The listing builds one solid part. Answer for the finished solid, in the listing's coordinates (mm). A direction names the side the tool comes from. Coordinates: 2 decimals unless noted, no trailing zeros. Order: outer loops, then holes, each group sorted by start corner. A loop starts at its lowest first (then second) coordinate and runs counter-clockwise, first axis right, second up. Notation, with made-up numbers: M -39.5,-7.5 L 10.5,-7.5 A14 cw 10.5,9.5 Z; hole C 19,39.5 d4. An arc over 180 degrees is marked long. One line per item, written item: value. Start each with the question number.
Q1. Straight lines are drawn through the part: line 1 along Z through (x, y) = (0, 18); line 2 along Z through (x, y) = (492.5, -41); line 3 along Y through (x, z) = (147, 80). For each, find the intervals that lie inside material, in ascending order. Write a range as [from, to].
Q2. The part is cut by section B-B on x = 23.5. Give the vertices of the cut face in (y, z).
Q3. The part is cut by section D-D on y = 47. Give the vertices of the cut face in (x, z).
Q4. The part is cut by section C-C on z = 87.5. Give the vertices of the cut face in (x, y).
Q5. Each of these flat-tipped pins is pushed along its axis until it touches: pin 1 Ø5 at (x, y) = (376, -54.5) entering from -Z; pin 2 Ø4 at (x, z) = (119, 162) entering from -Y; pin 3 Ø14 at (y, z) = (-71.5, 242) entering from -X. Where does it stop, or does it pass through?
Q6. For faces 1 (the flat face through (627.074, -38, 258)), 2 (the cylindrical face through (-287.495, -0.889, 347.275)), determine the directions among +Z, -Z, +X, -X, +Y, -Y from which every point of the face is accessible in a straight line to the end or side of a thin tool.
Q7. The part is cut by section A-A on y = -22.5. Give the vertices of the cut face in (x, z), then the cut area to 3 significant figures.
```python
from build123d import *

# Parameters (mm, degrees)
F2_DEPTH = 63.5
F0_W     = 627.0736455917
F0_H     = 80.0375938416
F3_DEPTH = 76.2
F5_D     = 17.5
F6_W     = 63.5
F6_H     = 80.0375938416
F7_DEPTH = 839.2885923386


with BuildPart() as f2:
    # F1 (on face) → F2 (new body, symmetric)
    with BuildSketch(Plane.XZ):
        with BuildLine():
            Line((0, 298.9611625671), (291.8738404898, 298.9611625671))
            ThreePointArc((291.8738404898, 298.9611625671), (-289.3594591256, 335.1473667086), (281.2837032222, 218.9235687256))
            Line((281.2837032222, 218.9235687256), (0, 218.9235687256))
            Line((0, 218.9235687256), (0, 298.9611625671))
        make_face()
    extrude(amount=F2_DEPTH, both=True)

    # F0 (on Front) → F3 (join)
    with BuildSketch(Plane.XZ):
        with Locations((313.5368227959, 258.9423656464)):
            Rectangle(F0_W, F0_H)
    extrude(amount=F3_DEPTH)

    # F5 (through all)
    with Locations(Plane(origin=(0, 63.5, 0), x_dir=(-1, 0, 0), z_dir=(0, 1, 0))):
        with Locations((0, 402.5558233261)):
            Hole(F5_D / 2)

    # F6 (on face) → F7 (join)
    with BuildSketch(Plane.YZ):
        with Locations((31.75, 258.9423656464)):
            Rectangle(F6_W, F6_H)
    extrude(amount=F7_DEPTH)


solid = f2.part
```
Output:
1. line 1: z = [4.98, 393.81], [411.31, 588.74]
1. line 2: z = [218.92, 298.96]
1. line 3: y = [-63.5, 63.5]
2. outline: M -76.2,218.92 L -63.5,218.92 L -63.5,5.93 L 63.5,5.93 L 63.5,587.79 L -63.5,587.79 L -63.5,298.96 L -76.2,298.96 Z
3. outline: M 281.28,218.92 L 839.29,218.92 L 839.29,298.96 L 291.87,298.96 A291.88 ccw long Z; hole C 0,402.56 d17.5
4. outline: M -203.38,-63.5 L 203.38,-63.5 L 203.38,63.5 L -203.38,63.5 Z
5. pin 1: stops at z = 218.92
5. pin 2: stops at y = -63.5
5. pin 3: stops at x = 0
6. face 1: +Z, -Z, +X, -Y
6. face 2: +Y, -Y
7. outline: M 281.28,218.92 L 627.07,218.92 L 627.07,298.96 L 291.87,298.96 A291.88 ccw long Z; hole C 0,402.56 d17.5
7. area: 295,000 mm^2
